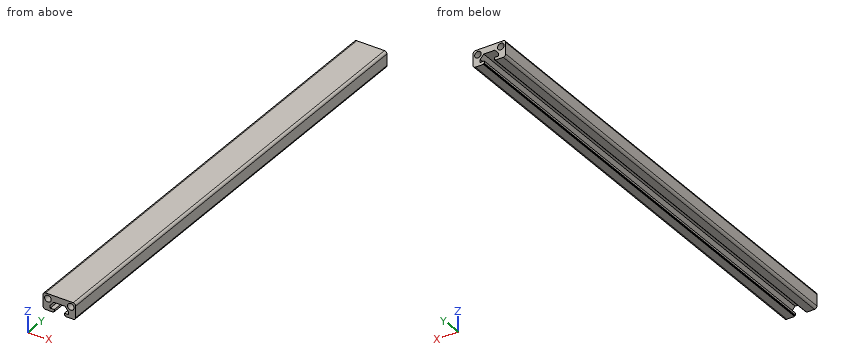
```python
from build123d import *

# Parameters (mm, degrees)
SKETCH_1_R      = 2
EXTRUDE_1_DEPTH = 288
FILLET_1_R      = 1.5


with BuildPart() as part:
    # 草图1 → 凸台-拉伸1 (new body)
    with BuildSketch(Plane(origin=(0, 0, 0), x_dir=(1, 0, 0), z_dir=(0, 1, 0))):
        Polygon((0, 0), (20, 0), (20, 10), (13.65, 10), (13.65, 9.510427602), (13.1, 9.510427602), (13.1, 8.2), (15.6, 8.2), (15.6, 6.447507136), (13.412706863, 3.9), (6.587293137, 3.9), (4.4, 6.447507136), (4.4, 8.2), (6.9, 8.2), (6.9, 9.510427602), (6.35, 9.510427602), (6.35, 10), (0, 10), align=None)
        with Locations(Location((3, 3, 0), (0, 0, 270))):
            Circle(SKETCH_1_R, mode=Mode.SUBTRACT)
        with Locations(Location((17, 3, 0), (0, 0, 270))):
            Circle(SKETCH_1_R, mode=Mode.SUBTRACT)
    extrude(amount=EXTRUDE_1_DEPTH)

    # 圆角1
    fillet_1_edges = [part.edges().sort_by_distance(p)[0] for p in [
        (0, 144, -10),
        (20, 144, -10),
        (20, 144, 0),
        (0, 144, 0),
    ]]
    fillet(fillet_1_edges, radius=FILLET_1_R)


solid = part.part
```
The listing builds one solid part. Answer for the finished solid, in the listing's coordinates (mm). Give positions to 0.01 mm unless a question says otherwise; leave off trailing zeros. Order: outer loops, then holes, each group sorted by start corner. A loop starts at its lowest first (then second) coordinate and runs counter-clockwise, first axis right, second up. Notation, with made-up numbers: (66.5, -38) - (86.5, -38) arc R19 cw to (86.5, -23) - close; hole circle Ø4 at (50, 50.25). An arc over 180 degrees is marked (long way). Answer in a Markdown table with one row per item. Add a question column.
Q1. Given P1, Ø0.7, axis at y = 211, z = -9, coming from the -X side; P2, Ø1, axis at x = 7, y = 153.5, coming from the -Z side; P3, Ø3.5, axis at x = 10.5, y = 132, coming from the -Z side; P4, Ø3, axis at x = 3, z = -3, coming from the -Y side, each flat-ended and moving along its own axis, determine where each tip first touches the part or whether it passes through.
Q2. The part is cut by section A-A (y = 228.5). Determine the outline of the cut face in (x, z), then the cut area to 3 significant figures.
Q3. Find the intervals of material crossed by line 1 along X through (y, z) = (160, -3); line 2 along X through (y, z) = (82, -8); line 3 along X through (y, z) = (28, -4.25), in increasing order. Write a range as [from, to].
Determined:
| question | item | result |
|---|---|---|
| 1 | P1 | stops at x = 0.01 |
| 1 | P2 | stops at z = -9.51 |
| 1 | P3 | stops at z = -3.9 |
| 1 | P4 | passes through |
| 2 | outline | (0, -8.5) arc R1.5 ccw to (1.5, -10) - (6.35, -10) - (6.35, -9.51) - (6.9, -9.51) - (6.9, -8.2) - (4.4, -8.2) - (4.4, -6.45) - (6.59, -3.9) - (13.41, -3.9) - (15.6, -6.45) - (15.6, -8.2) - (13.1, -8.2) - (13.1, -9.51) - (13.65, -9.51) - (13.65, -10) - (18.5, -10) arc R1.5 ccw to (20, -8.5) - (20, -1.5) arc R1.5 ccw to (18.5, 0) - (1.5, 0) arc R1.5 ccw to (0, -1.5) - close; hole circle Ø4 at (3, -3); hole circle Ø4 at (17, -3) |
| 2 | area | 119 mm² |
| 3 | line 1 | x = [0, 1], [5, 15], [19, 20] |
| 3 | line 2 | x = [0, 4.4], [15.6, 20] |
| 3 | line 3 | x = [0, 1.44], [4.56, 6.29], [13.71, 15.44], [18.56, 20] |
